Can you work these out from the model? Positions are in its coordinate system, mm. Round coordinates to 2 decimals unless told otherwise and drop trailing zeros. Loops run counter-clockwise (first coordinate to the right, second up) from the corner with the lowest first, then second, coordinate; pieces in that order, holes last. Notation, with made-up numbers: (47.5, -32.75) -> (56.5, -32.75) arc R20 ccw to (56.5, -18.75) -> close; hole circle Ø3 at (21, 2). An arc over 180 degrees is marked (long way). Write item = value, one per line.
from build123d import *

# Parameters (mm, degrees)
F0_W     = 76.5
F0_H     = 100
F1_DEPTH = 25.4
F2_R     = 5
F3_DEPTH = 76.501
F5_DEPTH = 76.501


with BuildPart() as f1:
    # F0 (on Top) → F1 (new body)
    with BuildSketch(Plane.XY):
        with Locations((0, 20)):
            Rectangle(F0_W, F0_H)
    extrude(amount=F1_DEPTH)

    # F2 (on face) → F3 (cut, through all)
    with BuildSketch(Plane.YZ.offset(38.25)):
        with Locations((-17.3, 15.875)):
            Circle(F2_R)
    extrude(amount=-F3_DEPTH, mode=Mode.SUBTRACT)

    # F4 (on face) → F5 (cut, through all)
    with BuildSketch(Plane.YZ.offset(38.25)):
        with BuildLine():
            ThreePointArc((-8.508814, 11.775603), (-6.43921, 7.57886), (-2.789891, 10.507748))
            ThreePointArc((-2.789891, 10.507748), (-5.140572, 13.436636), (-8.508814, 11.775603))
        make_face()
    extrude(amount=-F5_DEPTH, mode=Mode.SUBTRACT)


solid = f1.part
1. I need wall thicknesses on line 1 (Z direction, x = 15, y = -17); line 2 (Z direction, x = -23, y = -3.5); line 3 (Y direction, x = 8, z = 17.75). Which ranges of each line are inside material? Lowest first, please. Write a range as [from, to].
Entries:
line_1 = [0, 10.88], [20.87, 25.4]
line_2 = [0, 8.57], [12.45, 25.4]
line_3 = [-30, -21.94], [-12.66, 70]
2. I'm going to push a flat-ended pin straight in: pin 1 (8 mm diameter, centred on x = -6.5, y = -3.5, fed in from -Z). Where does the tip first touch, or does it pass through?
Entries:
pin_1 = 0
3. We'd pull the mould along Z, two halves only. Please class faces 1 (the cylindrical face through (0.535, -18.384, 10.994)), 2 (the flat face through (-1, 21, 25.4)), 3 (the flat face through (-1, -30, 13)): released by +Z, released by -Z, zero draft, split by the parting line, or undercut.
Entries:
face_1 = undercut
face_2 = released by +Z
face_3 = zero draft
4. Suppose I cut it at B-B, the plane x = 16.5. List the corners of the cut face in (y, z) for me (3 decimals), and give its area (3 significant figures).
Entries:
outline = (-30, 0) -> (70, 0) -> (70, 25.4) -> (-30, 25.4) -> close; hole circle Ø10 at (-17.3, 15.875); hole circle Ø6 at (-5.79, 10.508)
area = 2,430 mm²
5. Suppose I cut it at C-C, the plane y = -5. List the corners of the cut face in (x, z) for me, and give its area (3 significant figures).
Entries:
outline = (-38.25, 0) -> (38.25, 0) -> (38.25, 7.61) -> (-38.25, 7.61) -> close; (-38.25, 13.4) -> (38.25, 13.4) -> (38.25, 25.4) -> (-38.25, 25.4) -> close
area = 1,500 mm²
6. Suppose I cut it at A-A, the plane y = -17.3. List the corners of the cut face in (x, z) for me (3 decimals).
Entries:
outline = (-38.25, 0) -> (38.25, 0) -> (38.25, 10.875) -> (-38.25, 10.875) -> close; (-38.25, 20.875) -> (38.25, 20.875) -> (38.25, 25.4) -> (-38.25, 25.4) -> close
